Study the drawing (mm; zero at the part's minimum x, y, z) and answer. A direction names the side the tool comes from. Coordinates: 2 decimals unless noted, no trailing zeros. Order: outer loops, then holes, each group sorted by start corner. A loop starts at its lowest first (then second) coordinate and runs counter-clockwise, first axis right, second up. Notation, with made-up numbers: (-11.5, 69.25) -> (5.5, 69.25) arc R31 ccw to (5.5, 101.25) -> close; hole circle Ø9 at (9.25, 8.5). An arc over 180 degrees is marked (long way). One line per question, with ' | ' between items.
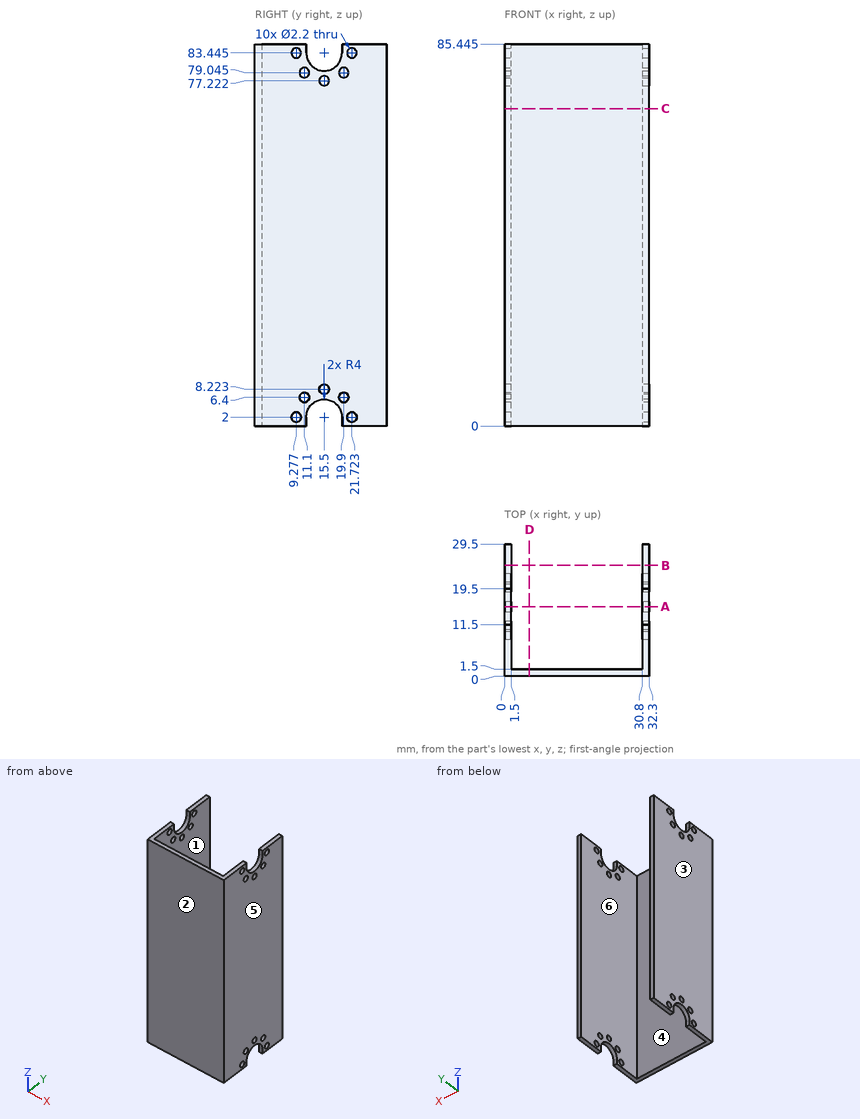
Item 1: Section C-C, the plane z = 71 is taken. Give the vertices of the cut face in (x, y).
Computed values:
outline: (0, 0) -> (32.3, 0) -> (32.3, 29.5) -> (30.8, 29.5) -> (30.8, 1.5) -> (1.5, 1.5) -> (1.5, 29.5) -> (0, 29.5) -> close
Item 2: Section B-B, the plane y = 24.75 is taken. Give the vertices of the cut face in (x, z) (1 decimal).
Computed values:
outline: (0, 0) -> (1.5, 0) -> (1.5, 85.4) -> (0, 85.4) -> close; (30.8, 0) -> (32.3, 0) -> (32.3, 85.4) -> (30.8, 85.4) -> close
Item 3: This flat-tipped pin is pushed along its axis until it touches: pin 1 Ø1.3 at (y, z) = (19.9, 79.045) entering from +X. Where does it stop, or does it pass through?
Computed values:
pin 1: passes through
Item 4: Section D-D, the plane x = 5.5 is taken. Give the vertices of the cut face in (y, z) (1 decimal).
Computed values:
outline: (0, 0) -> (1.5, 0) -> (1.5, 85.4) -> (0, 85.4) -> close
Item 5: Find the intervals of material crossed by L1, parallel to Z at x = 0.85, y = 11.1 (1 decimal); L2, parallel to X at y = 14, z = 70.5; L3, parallel to Y at x = 10, z = 11, in increasing order.
Computed values:
L1: z = 0 to 5.3, 7.5 to 77.9, 80.1 to 85.4 | L2: x = 0 to 1.5, 30.8 to 32.3 | L3: y = 0 to 1.5
Item 6: Determine the mould class of the marked faces 3, 4, 5 and 6 for opening direction X: pulls with the +X half, pulls with the -X half, needs draft (parallel to the pull), parting line crosses it, or undercut.
Computed values:
face 3: pulls with the -X half | face 4: undercut | face 5: pulls with the +X half | face 6: undercut
Item 7: For the marked faces 1 and 2, determine the directions among +Z, -Z, +X, -X, +Y, -Y from which every point of the face is accessible in a straight line to the end or side of a thin tool.
Computed values:
face 1: +Z, -Z, +Y | face 2: +Z, -Z, +X, -X, -Y
Item 8: Section A-A, the plane y = 15.5 is taken. Give the vertices of the cut face in (x, z) (1 decimal), plus the area to 3 significant figures.
Computed values:
outline: (0, 6) -> (1.5, 6) -> (1.5, 7.1) -> (0, 7.1) -> close; (0, 9.3) -> (1.5, 9.3) -> (1.5, 76.1) -> (0, 76.1) -> close; (0, 78.3) -> (1.5, 78.3) -> (1.5, 79.4) -> (0, 79.4) -> close; (30.8, 6) -> (32.3, 6) -> (32.3, 7.1) -> (30.8, 7.1) -> close; (30.8, 9.3) -> (32.3, 9.3) -> (32.3, 76.1) -> (30.8, 76.1) -> close; (30.8, 78.3) -> (32.3, 78.3) -> (32.3, 79.4) -> (30.8, 79.4) -> close | area: 207 mm^2
